Read the model definition and answer for the solid it produces. Units are mm, in the model's axes. A direction names the side the tool comes from. Coordinates: 2 decimals unless noted, no trailing zeros. Loops run counter-clockwise (first coordinate to the right, second up) from the corner with the lowest first, then second, coordinate; pieces in that order, holes last. Notation, with made-up numbers: M -19,72.25 L -13,72.25 A12 ccw -13,82.25 Z; hole C 11,-36.75 d4. An arc over 180 degrees is marked long. Put each result on its own line as item: value.
Autodesk Inventor part; units mm, degrees
ref_plane "YZ Plane" through (0, 0, 0) normal (1, 0, 0) x (0, 1, 0)
ref_plane "XZ Plane" through (0, 0, 0) normal (0, 1, 0) x (-1, 0, 0)
ref_plane "XY Plane" through (0, 0, 0) normal (0, 0, 1) x (1, 0, 0)
sketch "草圖1" plane through (0, 0, 0) normal (0, 1, 0) x (-1, 0, 0)
  circle A0 centre (0, 0) radius 3
  dimension "d0" = 6
extrude "擠出1" add sketch "草圖1" along normal blind 20
thread "螺紋1"
sketch "草圖2" plane through (0, 20, 0) normal (0, 1, 0) x (1, 0, 0)
  circle A0 centre (0, 0) radius 5
  dimension "d5" = 10
extrude "擠出2" add sketch "草圖2" along normal blind 4
sketch "草圖3" plane through (0, 24, 0) normal (0, 1, 0) x (1, 0, 0)
  line L0 (0, 2.7818) -> (2.4091, 1.3909)
  line L1 (2.4091, 1.3909) -> (2.4091, -1.3909)
  line L2 (2.4091, -1.3909) -> (0, -2.7818)
  line L3 (0, -2.7818) -> (-2.4091, -1.3909)
  line L4 (-2.4091, -1.3909) -> (-2.4091, 1.3909)
  line L5 (-2.4091, 1.3909) -> (0, 2.7818)
  point P0 (0, 0)
  point P1 (0, 0)
extrude "擠出3" cut sketch "草圖3" against normal blind 3
properties part number "M6screw"
1) Straight lines are drawn through the part: line 1 (Z direction, x = 0, y = 6.5); line 2 (Y direction, x = -3.75, z = -0.75); line 3 (X direction, y = 22, z = 0.25). For each, find the intervals that lie inside material, in ascending order. Write a range as [from, to].
Answer list:
line 1: z = [-3, 3]
line 2: y = [20, 24]
line 3: x = [-4.99, -2.41], [2.41, 4.99]
2) Find section D-D, the plane z = 2. Write down the section's boundary in (x, y).
Answer list:
outline: M -4.58,20 L -2.24,20 L -2.24,0 L 2.24,0 L 2.24,20 L 4.58,20 L 4.58,24 L 1.35,24 L 1.35,21 L -1.35,21 L -1.35,24 L -4.58,24 Z
3) Find section C-C, the plane x = -4. Write down the section's boundary in (y, z).
Answer list:
outline: M 20,-3 L 24,-3 L 24,3 L 20,3 Z
4) Find section A-A, the plane z = 0. Write down the section's boundary in (x, y).
Answer list:
outline: M -5,20 L -3,20 L -3,0 L 3,0 L 3,20 L 5,20 L 5,24 L 2.41,24 L 2.41,21 L -2.41,21 L -2.41,24 L -5,24 Z
5) Given pin 1 Ø6 at (y, z) = (7, -0.5) entering from +X; pin 2 Ø5 at (x, y) = (-2, 3) entering from -Z; pin 3 Ø4 at (x, y) = (3.5, 3.5) entering from -Z, each flat-ended and moving along its own axis, determine where each tip first touches the part or whether it passes through.
Answer list:
pin 1: stops at x = 3
pin 2: stops at z = -3
pin 3: stops at z = -2.6
6) Determine the mould class of faces 4 (the flat face through (-1.188, 22.521, 2.096)), 5 (the cylindrical face through (3, 10, 0)), 6 (the flat face through (-1.2, 24, -2.3)) for opening direction Z: released by +Z, released by -Z, zero draft, split by the parting line, or undercut.
Answer list:
face 4: undercut
face 5: split by the parting line
face 6: zero draft
7) Find section B-B, the plane y = 5. Write down the section's boundary in (x, z), plus the area to 3 significant figures.
Answer list:
outline: C 0,0 d6
area: 28.3 mm^2
8) Which of the six approach directions +Z, -Z, +X, -X, +Y, -Y give full straight-line access (tool end or side, diameter ignored) to faces 1 (the flat face through (0, 0, 0)), 2 (the flat face through (3.3, 20, -0.1)), 3 (the flat face through (2.409, 23, 0))?
Answer list:
face 1: +Z, -Z, +X, -X, -Y
face 2: -Y
face 3: +Y
